Verification items for this drawing (mm, ordinates from the low corner). Coordinates: 2 decimals unless noted, no trailing zeros. Order: outer loops, then holes, each group sorted by start corner. A loop starts at its lowest first (then second) coordinate and runs counter-clockwise, first axis right, second up. Notation, with made-up numbers: M 0,33.5 L 31,33.5 A14 ccw 31,39.5 Z; hole C 18.25,38 d8. An arc over 180 degrees is marked long. Write item = value, one per line.
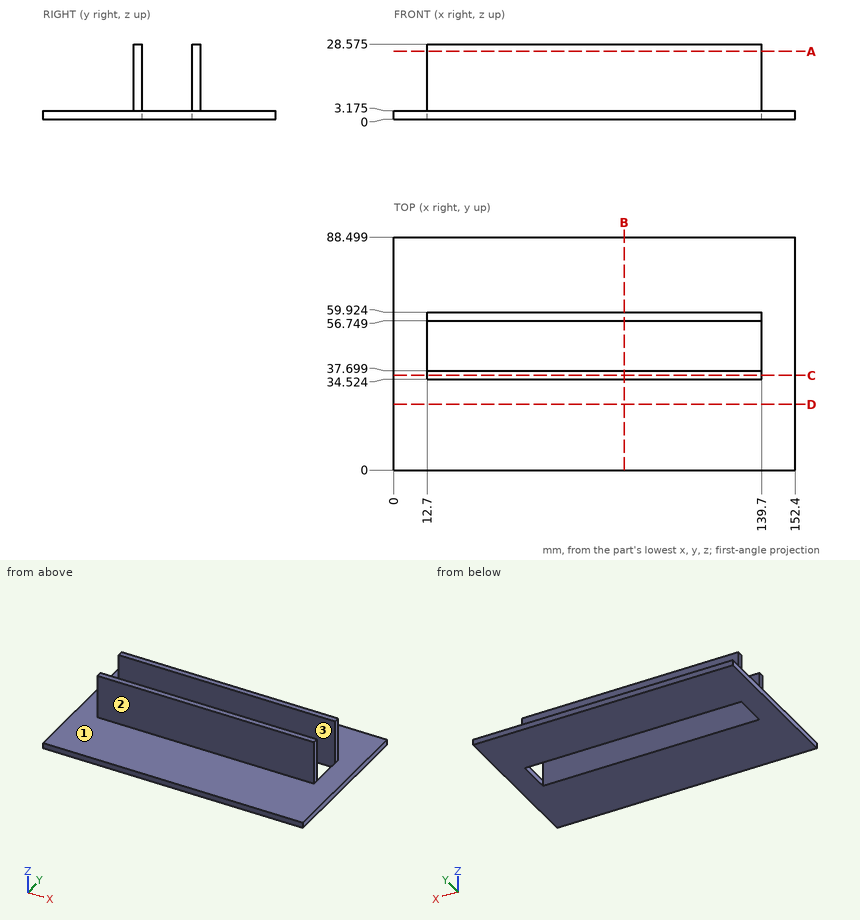
Item 1: Sectioned sample at B-B, the plane x = 87.5. Enter the section's corners in (y, z) (1 decimal).
Report:
outline = M 0,0 L 37.7,0 L 37.7,28.6 L 34.5,28.6 L 34.5,3.2 L 0,3.2 Z; M 56.7,0 L 88.5,0 L 88.5,3.2 L 59.9,3.2 L 59.9,28.6 L 56.7,28.6 Z
Item 2: Gauge pin test, flat ends, axial feed: pin 1 (8 mm diameter, centred on x = 70, z = 18, fed in from -Y); pin 2 (1.6 mm diameter, centred on y = 59, z = 14.5, fed in from -X); pin 3 (2 mm diameter, centred on x = 75.5, z = 20, fed in from +Y). Record the tip position at first contact, or that the pin passes through.
Report:
pin_1 = 34.52
pin_2 = 12.7
pin_3 = 59.92
Item 3: Release check for a two-part mould opening along Y. For the marked faces 1, 2 and 3 record: pulls with the +Y half, pulls with the -Y half, needs draft (parallel to the pull), parting line crosses it, or undercut.
Report:
face_1 = needs draft
face_2 = pulls with the -Y half
face_3 = undercut
Item 4: Scan lines: L1, parallel to Y at x = 86, z = 14.5; L2, parallel to X at y = 57.5, z = 8; L3, parallel to Z at x = 30.5, y = 63 (1 decimal). Record each from-to range of solid material in increasing order. Write a range as from..to.
Report:
L1 = 34.52..37.7, 56.75..59.92
L2 = 12.7..139.7
L3 = 0..3.2
Item 5: Sectioned sample at A-A, the plane z = 25.75. Enter the section's corners in (x, y).
Report:
outline = M 12.7,34.52 L 139.7,34.52 L 139.7,37.7 L 12.7,37.7 Z; M 12.7,56.75 L 139.7,56.75 L 139.7,59.92 L 12.7,59.92 Z
Item 6: Sectioned sample at C-C, the plane y = 36. Enter the section's corners in (x, z) (1 decimal), then the cut area to 3 significant figures.
Report:
outline = M 0,0 L 152.4,0 L 152.4,3.2 L 139.7,3.2 L 139.7,28.6 L 12.7,28.6 L 12.7,3.2 L 0,3.2 Z
area = 3,710 mm^2
Item 7: Sectioned sample at D-D, the plane y = 25. Enter the section's corners in (x, z) (1 decimal), then the cut area to 3 significant figures.
Report:
outline = M 0,0 L 152.4,0 L 152.4,3.2 L 0,3.2 Z
area = 484 mm^2
